Geometry check sheet. Reference: the model listing, model coordinates, mm. Round coordinates to 2 decimals unless told otherwise and drop trailing zeros. Write each loop counter-clockwise with the first axis right and the second up, starting at its lowest first coordinate (ties: lowest second). Pieces come first, ordered by that corner, then holes. Notation, with made-up numbers: M -25.75,54.5 L 8.25,54.5 A10 ccw 8.25,69.5 Z; hole C 55.25,41 d3. An arc over 180 degrees is marked long. One line per item, written item: value. Start each with the question number.
1. Section check C-C (z = 170.5). Record the boundary of the cut face in (x, y), and give its area (3 significant figures).
2. Scan lines: probe 1 along X at (y, z) = (0, 71); probe 2 along Y at (x, z) = (3.5, 142); probe 3 along Y at (x, z) = (131, 216.5). Record each from-to range of solid material in increasing order. Write a range as [from, to].
3. Depth check by flat-ended pin: P1, Ø3, axis at x = -38.5, z = 175, coming from the -Y side; P2, Ø1, axis at y = 91.5, z = 44.5, coming from the -X side; P3, Ø2, axis at y = 123.5, z = 121, coming from the +X side. Enter the tip coordinate at first touch or a pass-through.
4. Section check D-D (z = 282). Record the boundary of the cut face in (x, y).
Autodesk Inventor part; units mm, degrees
ref_plane "YZ Plane" through (0, 0, 0) normal (1, 0, 0) x (0, 1, 0)
ref_plane "XZ Plane" through (0, 0, 0) normal (0, 1, 0) x (-1, 0, 0)
ref_plane "XY Plane" through (0, 0, 0) normal (0, 0, 1) x (1, 0, 0)
sketch "Sketch1" plane through (0, 0, 0) normal (0, 0, 1) x (1, 0, 0)
  circle A0 centre (0, 0) radius 336.55
  circle A1 centre (0, 0) radius 368.3
  dimension "d0" = 673.1
  dimension "d1" = 736.6
extrude "Extrusion1" add sketch "Sketch1" along normal blind 304.8
sketch "Sketch2" plane through (0, 0, 304.8) normal (0, 0, 1) x (1, 0, 0)
  circle A0 centre (0, 0) radius 368.3
  circle A1 centre (0, 0) radius 371.221
  circle A2 centre (0, 0) radius 374.396
  dimension "d4" = 742.442
  dimension "d5" = 748.792
extrude "Extrusion2" add sketch "Sketch2" against normal blind 50.8 contours A1
extrude "Extrusion3" add sketch "Sketch2" against normal blind 25.4 contours A2
chamfer "Chamfer1" distance 2.921 angle 45 1 edges at (-368.3, 0, 254)
sketch "Sketch3" plane through (0, 0, 0) normal (0, 0, -1) x (-1, 0, 0)
  circle A0 centre (0, 0) radius 355.346
  circle A1 centre (0, 0) radius 336.55
  dimension "d13" = 710.692
extrude "Extrusion4" add sketch "Sketch3" along normal blind 12.7
fillet "Fillet1" radius 0.7937 2 edges at (355.346, 0, 0) (-371.221, 0, 279.4)
chamfer "Chamfer2" distance 0.7937 angle 45 1 edges at (355.346, 0, -12.7)
chamfer "Chamfer3" distance 0.7937 angle 45 1 edges at (-374.396, 0, 279.4)
sketch "Sketch4" plane through (0, 0, 0) normal (1, 0, 0) x (0, 1, 0)
  line L0 (371.221, 278.6063) -> (371.221, 254) construction
  line L1 (-374.396, 304.8) -> (374.396, 304.8) construction
  line L2 (371.221, 273.05) -> (369.4409, 271.2699)
  arc A0 (369.4409, 271.2699) -> (368.046, 267.9023) centre (372.8085, 267.9023) ccw
  line L3 (368.046, 267.9023) -> (368.046, 267.0852)
  arc A1 (368.046, 267.0852) -> (369.4409, 263.7176) centre (372.8085, 267.0852) ccw
  line L4 (369.4409, 263.7176) -> (371.221, 261.9375)
  line L5 (371.221, 261.9375) -> (371.221, 273.05)
  line L6 (0, -76.2) -> (0, 368.3)
  point P0 (0, 0)
  dimension "d23" = 11.1125
  dimension "d24" = 3.175
  dimension "d25" = 4.7625
  dimension "d26" = 31.75
  dimension "d27" = 45
revolve "Revolution1" cut sketch "Sketch4" angle 360 about axis through (0, 0, -10) along (0, 0, 1)
sketch "Sketch5" plane through (0, 0, -12.7) normal (0, 0, -1) x (-1, 0, 0)
  circle A0 centre (0, 0) radius 336.55
  circle A1 centre (0, 0) radius 368.3
extrude "Extrusion5" add sketch "Sketch5" along normal blind 12.7 and the other way blind 12.7
sketch "Sketch6" plane through (0, 0, 304.8) normal (0, 0, 1) x (1, 0, 0)
  circle A0 centre (0, 0) radius 374.396
  circle A1 centre (0, 0) radius 336.55
  circle A2 centre (0, 0) radius 380.746
  dimension "d33" = 6.35
extrude "Extrusion6" add sketch "Sketch6" along normal blind 12.7 and the other way blind 50.8 contours A0 | A2
chamfer "Chamfer6" distance 9.525 angle 45 1 edges at (-380.746, 0, 254)
equation "\"d10\" = -0.5 * d1 + 0.5 * d4"
properties part number "A1-19037-100-06 HCWI liner - pup - as cast" material "Iron, HCWI"
Result sheet:
1. outline: C 0,0 d736.6; hole C 0,0 d673.1
1. area: 70,300 mm2
2. probe 1: x = [-368.3, -336.55], [336.55, 368.3]
2. probe 2: y = [-368.28, -336.53], [336.53, 368.28]
2. probe 3: y = [-344.21, -310.01], [310.01, 344.21]
3. P1: stops at y = -366.44
3. P2: stops at x = -356.88
3. P3: stops at x = 347.33
4. outline: C 0,0 d761.49; hole C 0,0 d673.1
